```python
from build123d import *

# Parameters (mm, degrees)
SKETCH_R        = 11.00074
PAD_DEPTH       = 6.4262
SKETCH001_R     = 4.67614
PAD001_DEPTH    = 3.175
SKETCH002_R     = 4.67614
PAD002_DEPTH    = 3.175
SKETCH003_R     = 2.06375
POCKET_DEPTH    = 12.7772
SKETCH004_R     = 1.20015
POCKET001_DEPTH = 9.6022


with BuildPart() as part:
    # Sketch → Pad (new body)
    with BuildSketch(Plane.XY):
        Circle(SKETCH_R)
    extrude(amount=PAD_DEPTH)

    # Sketch001 → Pad001 (new body)
    with BuildSketch(Plane.XY.offset(6.4262)):
        Circle(SKETCH001_R)
    extrude(amount=PAD001_DEPTH)

    # Sketch002 → Pad002 (new body)
    with BuildSketch(Plane(origin=(0, 0, 0), x_dir=(1, 0, 0), z_dir=(0, 0, -1))):
        Circle(SKETCH002_R)
    extrude(amount=PAD002_DEPTH)

    # Sketch003 → Pocket (cut, through all)
    with BuildSketch(Plane(origin=(0, 0, -3.175), x_dir=(1, 0, 0), z_dir=(0, 0, -1))):
        Circle(SKETCH003_R)
    extrude(amount=-POCKET_DEPTH, mode=Mode.SUBTRACT)

    # Sketch004 → Pocket001 (cut, through all)
    with BuildSketch(Plane(origin=(0, 0, 0), x_dir=(1, 0, 0), z_dir=(0, 0, -1))):
        with Locations((7.43331, 0)):
            Circle(SKETCH004_R)
        with Locations((0, -7.43331)):
            Circle(SKETCH004_R)
        with Locations((0, 7.43331)):
            Circle(SKETCH004_R)
        with Locations((-7.43331, 0)):
            Circle(SKETCH004_R)
    extrude(amount=-POCKET001_DEPTH, mode=Mode.SUBTRACT)


solid = part.part
```
Could you check a few things on this model? Use its own coordinates, in mm. A direction names the side the tool comes from. Round coordinates to 2 decimals unless told otherwise and drop trailing zeros. Write each loop counter-clockwise with the first axis right and the second up, starting at its lowest first coordinate (ties: lowest second). Pieces come first, ordered by that corner, then holes. Notation, with made-up numbers: M 24,41 L 69,41 A20 cw 69,49 Z; hole C -8.5,45.25 d9. An arc over 180 degrees is marked long. Write each question's results on one line, items separated by ' | '. Start each with the question number.
1. I need wall thicknesses on L1, parallel to Y at x = 0, z = 2; L2, parallel to Y at x = -0.5, z = 4.5; L3, parallel to Z at x = 2.75, y = -5.5. Which ranges of each line are inside material? Lowest first, please. Write a range as from..to.
2. On a 3-axis mill with a long thin cutter (end or side, diameter ignored), from which of +Z, -Z, +X, -X, +Y, -Y can I reach the whole of each face in a straight line? I mean faces 5 (the face through (-6.3, -0.4, 3.2)), 6 (the face through (0, -5, 6.426)), 7 (the face through (-0.609, -4.636, -1.565)). Say none if no direction works.
3. Imagine slicing it at C-C on x = 7.5. List the corners of the cut face in (y, z) for me, and give its area (3 significant figures).
4. Imagine slicing it at D-D on z = 7.25. List the corners of the cut face in (x, y) for me, and give its area (3 significant figures).
5. Imagine slicing it at A-A on y = 0. List the corners of the cut face in (x, z) for me (3 decimals).
6. I'm going to push flat-ended pins straight in: pin 1 Ø2 at (x, y) = (0, -7.43) entering from -Z; pin 2 Ø2 at (x, y) = (-8, -7.5) entering from -Z; pin 3 Ø6 at (y, z) = (1, 7) entering from -X; pin 4 Ø1 at (x, z) = (5.5, 4) entering from +Y. Where does each tip first touch, or does it pass through?
7. Thinking about a two-plate mould opening in X: for faces 1 (the face through (-0.609, 4.636, 7.991)), 2 (the face through (8.58, -0.36, 3.17)), 3 (the face through (-0.156, 6.243, 3.168)), 4 (the face through (0, -5, 0)), which applies, +X half, -X half, draft (parallel to the pull), parting line (faces both ways), or undercut?
Result sheet:
1) L1: y = -11..-8.63, -6.23..-2.06, 2.06..6.23, 8.63..11 | L2: y = -10.99..-8.52, -6.34..-2, 2..6.34, 8.52..10.99 | L3: z = 0..6.43
2) face 5: +Z, -Z | face 6: +Z | face 7: -Z
3) outline: M -8.05,0 L -1.2,0 L -1.2,6.43 L -8.05,6.43 Z; M 1.2,0 L 8.05,0 L 8.05,6.43 L 1.2,6.43 Z | area: 88.0 mm^2
4) outline: C 0,0 d9.35; hole C 0,0 d4.13 | area: 55.3 mm^2
5) outline: M -11.001,0 L -8.633,0 L -8.633,6.426 L -11.001,6.426 Z; M -6.233,0 L -4.676,0 L -4.676,-3.175 L -2.064,-3.175 L -2.064,9.601 L -4.676,9.601 L -4.676,6.426 L -6.233,6.426 Z; M 2.064,-3.175 L 4.676,-3.175 L 4.676,0 L 6.233,0 L 6.233,6.426 L 4.676,6.426 L 4.676,9.601 L 2.064,9.601 Z; M 8.633,0 L 11.001,0 L 11.001,6.426 L 8.633,6.426 Z
6) pin 1: passes through | pin 2: stops at z = 0 | pin 3: stops at x = -11 | pin 4: stops at y = 9.8
7) face 1: parting line | face 2: undercut | face 3: undercut | face 4: draft
